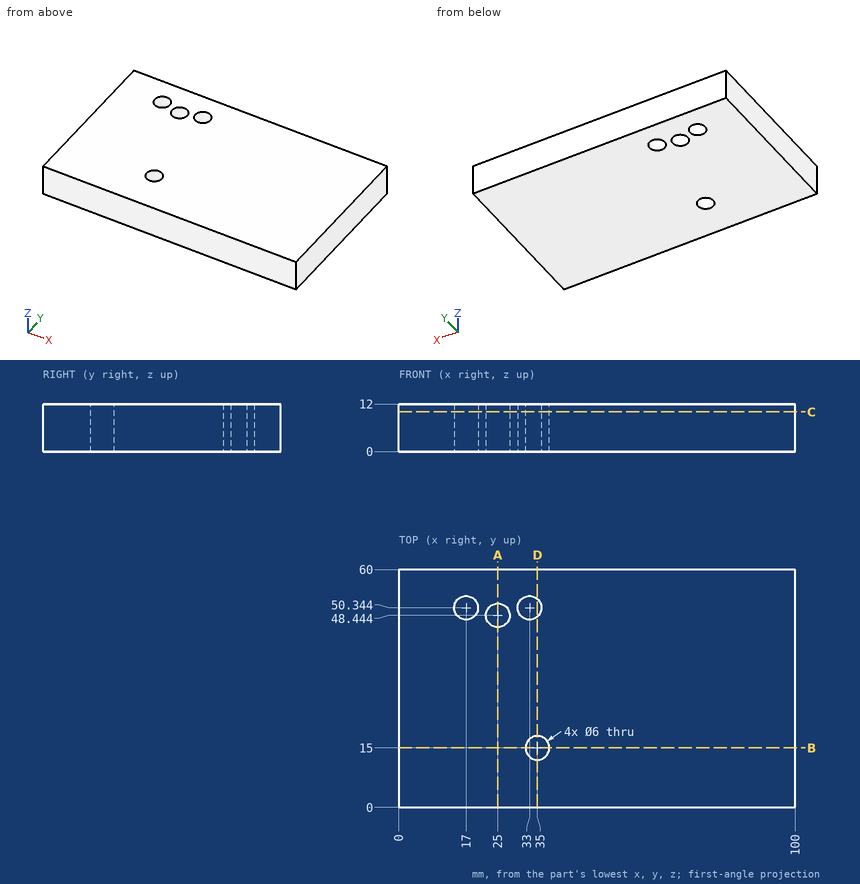
Design review of the part shown in the three views and the two pictorial views. Dimensions are in mm from the part's minimum x, y and z. Round coordinates to 2 decimals unless told otherwise and drop trailing zeros. Write each loop counter-clockwise with the first axis right and the second up, starting at its lowest first coordinate (ties: lowest second). Pieces come first, ordered by that corner, then holes.
Item 1: Clearance check with a flat-ended pin moving along its axis: pin 1 Ø5.5 at (x, y) = (25, 48.44) entering from +Z. State where the tip first meets the part, or that it passes through.
Item 2: For probe 1 along Y at (x, z) = (35, 4.75); probe 2 along X at (y, z) = (15, 3.25); probe 3 along Y at (x, z) = (25, 6), list the stretches that pass through material, from the lowest coordinate up.
Item 3: We need section A-A on x = 25. Write out the cut boundary in (y, z).
Item 4: We need section D-D on x = 35. Write out the cut boundary in (y, z).
Item 5: We need section B-B on y = 15. Write out the cut boundary in (x, z), and give its area (3 significant figures).
Item 6: We need section C-C on z = 10. Write out the cut boundary in (x, y), and give its area (3 significant figures).
Returned:
1. pin 1: passes through
2. probe 1: y = 0 to 12, 18 to 48.11, 52.58 to 60
2. probe 2: x = 0 to 32, 38 to 100
2. probe 3: y = 0 to 45.44, 51.44 to 60
3. outline: (0, 0) - (45.44, 0) - (45.44, 12) - (0, 12) - close; (51.44, 0) - (60, 0) - (60, 12) - (51.44, 12) - close
4. outline: (0, 0) - (12, 0) - (12, 12) - (0, 12) - close; (18, 0) - (48.11, 0) - (48.11, 12) - (18, 12) - close; (52.58, 0) - (60, 0) - (60, 12) - (52.58, 12) - close
5. outline: (0, 0) - (32, 0) - (32, 12) - (0, 12) - close; (38, 0) - (100, 0) - (100, 12) - (38, 12) - close
5. area: 1,130 mm2
6. outline: (0, 0) - (100, 0) - (100, 60) - (0, 60) - close; hole circle Ø6 at (17, 50.34); hole circle Ø6 at (25, 48.44); hole circle Ø6 at (33, 50.34); hole circle Ø6 at (35, 15)
6. area: 5,890 mm2
